Answer from the drawing. Dimensions are ordinates in mm from the lowest x, y and z of the part. A direction names the side the tool comes from. Give positions to 0.01 mm unless a question says otherwise; leave off trailing zeros. Order: outer loops, then holes, each group sorted by start corner. A loop starts at its lowest first (then second) coordinate and runs counter-clockwise, first axis right, second up.
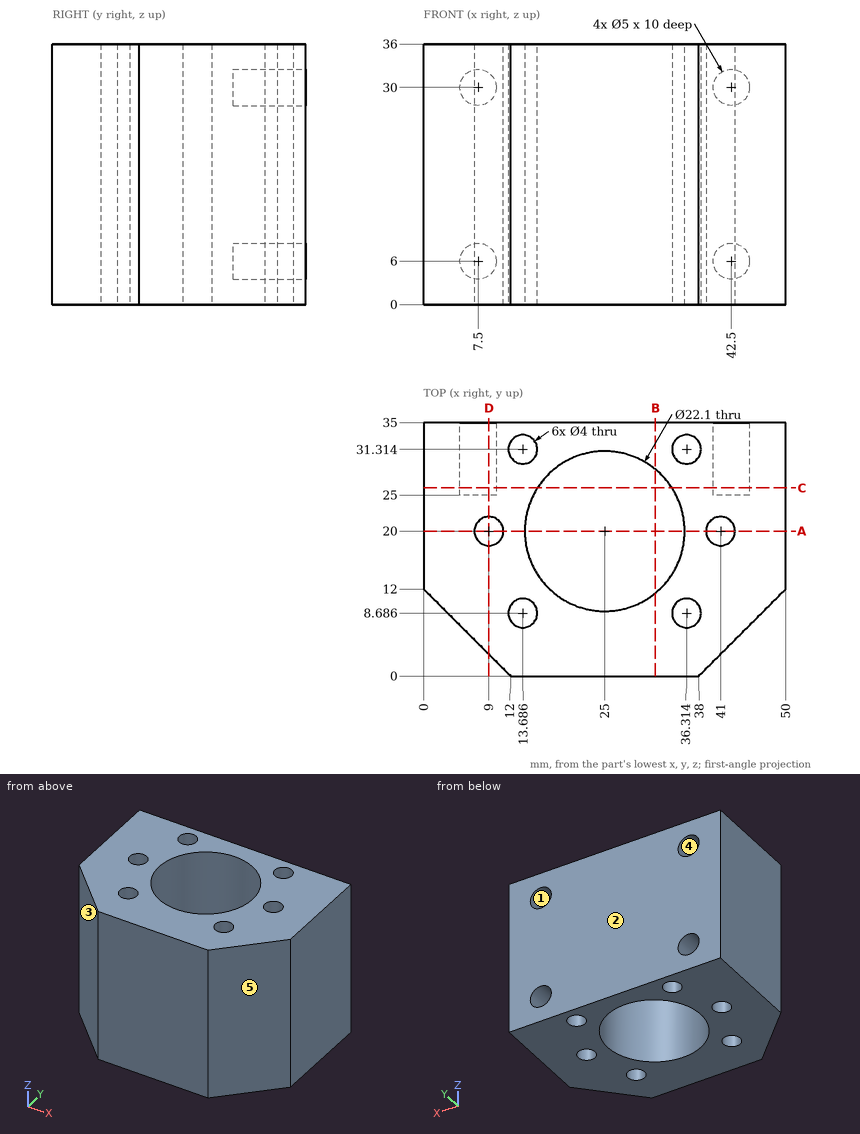
1) The part is cut by section B-B on x = 32. Determine the outline of the cut face in (y, z).
Final values:
outline: (0, 0) - (11.45, 0) - (11.45, 36) - (0, 36) - close; (28.55, 0) - (35, 0) - (35, 36) - (28.55, 36) - close
2) The part is cut by section C-C on y = 26. Determine the outline of the cut face in (x, z).
Final values:
outline: (0, 0) - (15.72, 0) - (15.72, 36) - (0, 36) - close; (34.28, 0) - (50, 0) - (50, 36) - (34.28, 36) - close; hole circle Ø5 at (7.5, 6); hole circle Ø5 at (7.5, 30); hole circle Ø5 at (42.5, 6); hole circle Ø5 at (42.5, 30)
3) For a pull along X with two mould halves and no side action, classify the marked faces 1, 2 and 3 as released by +X, released by -X, zero draft, split by the parting line, or undercut.
Final values:
face 1: undercut
face 2: zero draft
face 3: released by -X
4) A tool of negligible diameter and unlimited length cuts with its end or side. For the marked faces 4 and 5, from which of +Z, -Z, +X, -X, +Y, -Y can it reach the whole face along a straight path? Write none if from no direction.
Final values:
face 4: +Y
face 5: +Z, -Z, +X, -Y
5) The part is cut by section D-D on x = 9. Determine the outline of the cut face in (y, z), and give its area (3 significant figures).
Final values:
outline: (3, 0) - (18, 0) - (18, 36) - (3, 36) - close; (22, 0) - (35, 0) - (35, 4) - (25, 4) - (25, 8) - (35, 8) - (35, 28) - (25, 28) - (25, 32) - (35, 32) - (35, 36) - (22, 36) - close
area: 928 mm2
6) The part is cut by section A-A on y = 20. Determine the outline of the cut face in (x, z).
Final values:
outline: (0, 0) - (7, 0) - (7, 36) - (0, 36) - close; (11, 0) - (13.95, 0) - (13.95, 36) - (11, 36) - close; (36.05, 0) - (39, 0) - (39, 36) - (36.05, 36) - close; (43, 0) - (50, 0) - (50, 36) - (43, 36) - close
7) Consider L1, parallel to X at y = 31.5, z = 6 (1 decimal); L2, parallel to Y at x = 13, z = 6.5 (1 decimal); L3, parallel to Z at x = 7.5, y = 31. Determine where each line is inside the solid, lowest interval first.
Final values:
L1: x = 0 to 5, 10 to 11.7, 15.7 to 34.3, 38.3 to 40, 45 to 50
L2: y = 0 to 6.8, 10.6 to 29.4, 33.2 to 35
L3: z = 0 to 3.5, 8.5 to 27.5, 32.5 to 36
8) Given pin 1 (3 mm diameter, centred on x = 36.31, y = 8.69, fed in from -Z); pin 2 (3 mm diameter, centred on x = 42.5, z = 30, fed in from -Y); pin 3 (4.5 mm diameter, centred on x = 7.5, z = 6, fed in from -Y); pin 4 (1.5 mm diameter, centred on x = 8, z = 29, fed in from +Y), each flat-ended and moving along its own axis, determine where each tip first touches the part or whether it passes through.
Final values:
pin 1: passes through
pin 2: stops at y = 3
pin 3: stops at y = 2.25
pin 4: stops at y = 25
